Can you work these out from the drawing? Everything is in mm from the part's minimum corner. A direction names the side the tool comes from. Round coordinates to 2 decimals unless told otherwise and drop trailing zeros. Loops run counter-clockwise (first coordinate to the right, second up) from the corner with the lowest first, then second, coordinate; pieces in that order, holes last. Notation, with made-up numbers: (13, -8) - (62, -8) arc R17 ccw to (62, -1) - close; hole circle Ø3 at (-18, 71.25). An arc over 180 degrees is marked (long way). Answer as CSV lines item,"result". Start each with the question number.
1) Which directions (+Z, -Z, +X, -X, +Y, -Y) give clear straight access to the entire face, cutting with the end or side of a thin tool? Please do the marked faces 1 and 2.
2) Suppose I cut it at D-D, the plane x = 66.75. Write out the boundary of the cut face in (y, z), then the cut area to 3 significant figures.
3) Please list where these lines run through material, in increasing order: line 1 along X through (y, z) = (18.7, 24.15) (3 decimals); line 2 along Y through (x, z) = (45.5, 1.15); line 3 along Y through (x, z) = (54.5, 14).
4) Suppose I cut it at C-C, the plane y = 7.5. Write out the boundary of the cut face in (x, z), then the cut area to 3 significant figures.
5) Suppose I cut it at B-B, the plane x = 4.9. Write out the boundary of the cut face in (y, z) (3 decimals), then the cut area to 3 significant figures.
6) I'm going to push flat-ended pins straight in: pin 1 Ø5.5 at (x, z) = (86.1, 10.7) entering from -Y; pin 2 Ø3 at (x, z) = (67, 18.5) entering from +Y; pin 3 Ø10 at (y, z) = (13.5, 7.5) entering from -X; pin 4 Ø2 at (x, z) = (4.9, 10.7) entering from +Y. Where does each tip first touch, or does it pass through?
7) Suppose I cut it at A-A, the plane z = 10.7. Write out the boundary of the cut face in (x, y) (3 decimals), then the cut area to 3 significant figures.
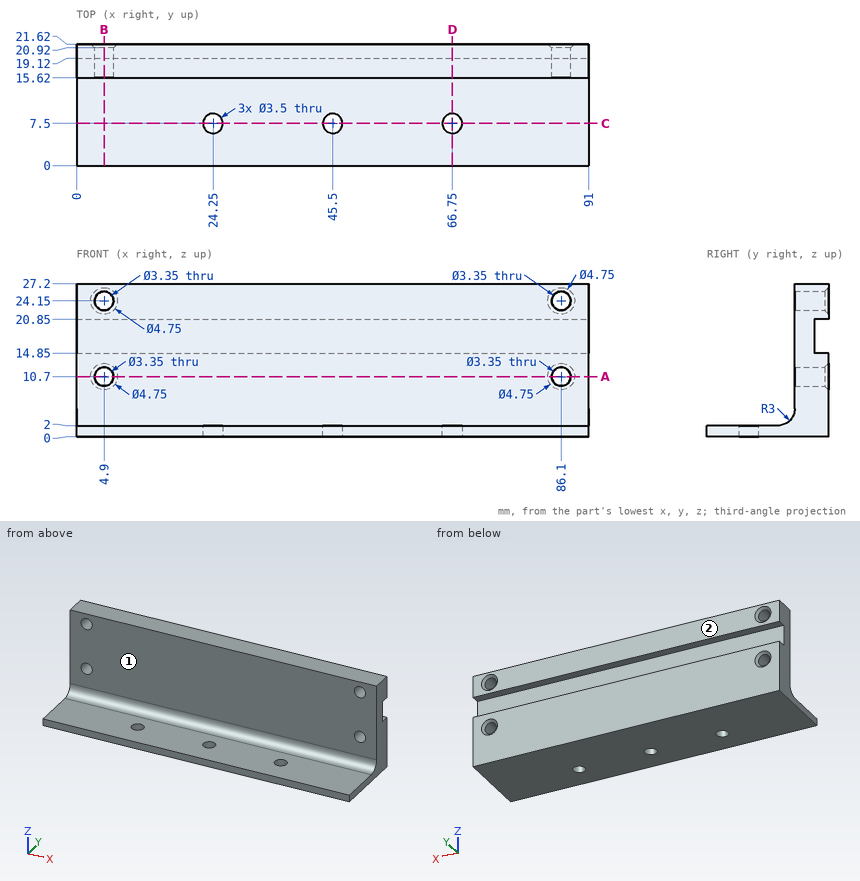
Filled sheet:
1,face 1,"+Z, +X, -X, -Y"
1,face 2,"+Z, -Z, +X, -X, +Y"
2,outline,"(0, 0) - (5.75, 0) - (5.75, 2) - (0, 2) - close; (9.25, 0) - (21.62, 0) - (21.62, 14.85) - (19.12, 14.85) - (19.12, 20.85) - (21.62, 20.85) - (21.62, 27.2) - (15.62, 27.2) - (15.62, 5) arc R3 cw to (12.62, 2) - (9.25, 2) - close"
2,area,"174 mm²"
3,line 1,"0 to 3.225, 6.575 to 84.425, 87.775 to 91"
3,line 2,"0 to 5.75, 9.25 to 21.62"
3,line 3,"15.62 to 21.62"
4,outline,"(0, 0) - (22.5, 0) - (22.5, 2) - (0, 2) - close; (26, 0) - (43.75, 0) - (43.75, 2) - (26, 2) - close; (47.25, 0) - (65, 0) - (65, 2) - (47.25, 2) - close; (68.5, 0) - (91, 0) - (91, 2) - (68.5, 2) - close"
4,area,"161 mm²"
5,outline,"(0, 0) - (21.62, 0) - (21.62, 8.325) - (20.92, 9.025) - (15.62, 9.025) - (15.62, 5) arc R3 cw to (12.62, 2) - (0, 2) - close; (15.62, 12.375) - (20.92, 12.375) - (21.62, 13.075) - (21.62, 14.85) - (19.12, 14.85) - (19.12, 20.85) - (21.62, 20.85) - (21.62, 21.775) - (20.92, 22.475) - (15.62, 22.475) - close; (15.62, 25.825) - (20.92, 25.825) - (21.62, 26.525) - (21.62, 27.2) - (15.62, 27.2) - close"
5,area,"140 mm²"
6,pin 1,"y = 15.62"
6,pin 2,"y = 19.12"
6,pin 3,"x = 0"
6,pin 4,"through"
7,outline,"(0, 15.62) - (3.225, 15.62) - (3.225, 20.92) - (2.525, 21.62) - (0, 21.62) - close; (6.575, 15.62) - (84.425, 15.62) - (84.425, 20.92) - (83.725, 21.62) - (7.275, 21.62) - (6.575, 20.92) - close; (87.775, 15.62) - (91, 15.62) - (91, 21.62) - (88.475, 21.62) - (87.775, 20.92) - close"
7,area,"505 mm²"
